Here's how the part is built. I have some questions about the finished solid (model axes, mm). A direction names the side the tool comes from. Give positions to 0.01 mm unless a question says otherwise; leave off trailing zeros. Loops run counter-clockwise (first coordinate to the right, second up) from the corner with the lowest first, then second, coordinate; pieces in that order, holes last. Notation, with made-up numbers: M 34,-16.5 L 62,-16.5 A11 ccw 62,1.5 Z; hole C 63.5,32 d1. An arc over 180 degrees is marked long. Answer as CSV lines item,"result". Start each with the question number.
Item 1: I want a section at B-B on z = 0. List the corners of the cut face in (x, y) for me, plus the area to 3 significant figures.
Item 2: Will these pins go through, and if not, where does the flat tip stop? P1, Ø1.2, axis at x = -6.5, y = 1.5, coming from the +Z side; P2, Ø1.5, axis at x = -32, y = 2, coming from the -Z side; P3, Ø2.5, axis at x = -38.5, z = 0, coming from the -Y side.
Item 3: I want a section at A-A on x = 38.5. List the corners of the cut face in (y, z) for me.
Item 4: If we mould it in two halves opening along Z, with no side actions, what happens to faces 4 (the cylindrical face through (-34.28, 1.97, 3.2)), 5 (the cylindrical face through (43.497, 1.972, -0.161)), 6 (the cylindrical face through (-37.3, 1.5, 0.9))? For each: released by +Z, released by -Z, zero draft, split by the parting line, or undercut.
Item 5: I want a section at C-C on x = -38.5. List the corners of the cut face in (y, z) for me, plus the area to 3 significant figures.
Item 6: For faces 1 (the cylindrical face through (34.28, 1.97, -3.2)), 2 (the flat face through (1, 4, 0)), 3 (the flat face through (0, 2, 3)), which set-ups out of +Z, -Z, +X, -X, +Y, -Y let a thin tool reach every point of the face, with its end or its side?
Item 7: If I drill on line 1 along X through (y, z) = (1.35, 0); line 2 along X through (y, z) = (2, 0.5); line 3 along Z through (x, y) = (-38.5, 1.55), over which ranges is the centre line in solid material (lowest first)? Write a range as from..to.
from build123d import *

# Parameters (mm, degrees)
SKETCH1_W                = 73.441671578
SKETCH1_H                = 6
BOSS_EXTRUDE1_DEPTH      = 4
SKETCH2_R                = 5
BOSS_EXTRUDE3_DEPTH      = 4
SKETCH3_R                = 5
BOSS_EXTRUDE4_DEPTH      = 4
FILLET1_R                = 3
FILLET3_R                = 3
F_3_0_3_DIAMETER_HOLE1_D = 3
F_6_0_6_DIAMETER_HOLE1_D = 6
CHAMFER1_SIZE            = 2
CHAMFER2_SIZE            = 1
FILLET4_R                = 0.5


with BuildPart() as part:
    # Sketch1 → Boss-Extrude1 (new body)
    with BuildSketch(Plane(origin=(0, 0, 0), x_dir=(1, 0, 0), z_dir=(0, 1, 0))):
        with Locations((1.782889385, 0)):
            Rectangle(SKETCH1_W, SKETCH1_H)
    extrude(amount=BOSS_EXTRUDE1_DEPTH)


with BuildPart() as body_2:
    # Sketch2 → Boss-Extrude3 (new body)
    with BuildSketch(Plane.XZ):
        with Locations(Location((38.5, 0, 0), (0, 0, 270))):
            Circle(SKETCH2_R)
    extrude(amount=-BOSS_EXTRUDE3_DEPTH)


with BuildPart() as body_3:
    # Sketch3 → Boss-Extrude4 (new body)
    with BuildSketch(Plane.XZ):
        with Locations(Location((-38.5, 0, 0), (0, 0, 270))):
            Circle(SKETCH3_R)
    extrude(amount=-BOSS_EXTRUDE4_DEPTH)


with BuildPart() as part_1:
    add(part.part)

    # Intersect3: read off the stored shape, not the designer's step
    # Intersect3: union body 3
    add(body_3.part)

    # Fillet1
    fillet1_edges = [part_1.edges().sort_by_distance(p)[0] for p in [
        (-34.5, 2, 3),
        (-34.5, 2, -3),
    ]]
    fillet(fillet1_edges, radius=FILLET1_R)

    # Intersect4: read off the stored shape, not the designer's step
    # Intersect4: union body 2
    add(body_2.part)

    # Fillet3
    fillet3_edges = [part_1.edges().sort_by_distance(p)[0] for p in [
        (34.5, 2, 3),
        (34.5, 2, -3),
    ]]
    fillet(fillet3_edges, radius=FILLET3_R)

    # Ø3.0 (3) Diameter Hole1 (through all)
    with Locations(Plane(origin=(0, 4, 0), x_dir=(1, 0, 0), z_dir=(0, 1, 0))):
        with Locations((-38.5, 0)):
            Hole(F_3_0_3_DIAMETER_HOLE1_D / 2)

    # Ø6.0 (6) Diameter Hole1 (through all)
    with Locations(Plane(origin=(0, 4, 0), x_dir=(1, 0, 0), z_dir=(0, 1, 0))):
        with Locations((38.5, 0)):
            Hole(F_6_0_6_DIAMETER_HOLE1_D / 2)

    # Chamfer1
    chamfer1_edges = [part_1.edges().sort_by_distance(p)[0] for p in [
        (-37, 4, 0),
    ]]
    chamfer(chamfer1_edges, length=CHAMFER1_SIZE)

    # Chamfer2
    chamfer2_edges = [part_1.edges().sort_by_distance(p)[0] for p in [
        (-37, 0, 0),
    ]]
    chamfer(chamfer2_edges, length=CHAMFER2_SIZE)

    # Fillet4
    fillet4_edges = [part_1.edges().sort_by_distance(p)[0] for p in [
        (41.5, 4, 0),
    ]]
    fillet(fillet4_edges, radius=FILLET4_R)


solid = part_1.part
Result:
1,outline,"M -43.5,0 L -41,0 L -40,1 L -40,2 L -42,4 L -43.5,4 Z; M -37,1 L -36,0 L 35.5,0 L 35.5,3.5 A0.5 ccw 35,4 L -35,4 L -37,2 Z; M 41.5,0 L 43.5,0 L 43.5,4 L 42,4 A0.5 ccw 41.5,3.5 Z"
1,area,"307 mm^2"
2,P1,"z = 3"
2,P2,"z = -3"
2,P3,"through"
3,outline,"M 0,-5 L 4,-5 L 4,-3.5 A0.5 ccw 3.5,-3 L 0,-3 Z; M 0,3 L 3.5,3 A0.5 ccw 4,3.5 L 4,5 L 0,5 Z"
4,face 4,"released by +Z"
4,face 5,"split by the parting line"
4,face 6,"undercut"
5,outline,"M 0,-5 L 4,-5 L 4,-3.5 L 2,-1.5 L 1,-1.5 L 0,-2.5 Z; M 0,2.5 L 1,1.5 L 2,1.5 L 4,3.5 L 4,5 L 0,5 Z"
5,area,"23.0 mm^2"
6,face 1,"-Z, +Y, -Y"
6,face 2,"+Z, -Z, +X, -X, +Y"
6,face 3,"+Z, +Y, -Y"
7,line 1,"-43.5..-40, -37..35.5, 41.5..43.5"
7,line 2,"-43.47..-39.91, -37.09..35.54, 41.46..43.47"
7,line 3,"-5..-1.5, 1.5..5"
